Read the model definition and answer for the solid it produces. Units are mm, in the model's axes. Face numbers are marked on the shaded views. A direction names the side the tool comes from. Coordinates: 2 decimals unless noted, no trailing zeros. Write each loop counter-clockwise with the first axis right and the second up, starting at its lowest first coordinate (ties: lowest second). Pieces come first, ordered by that corner, then holes.
Item 1: Section D-D (z = 1) is taken. Give the vertices of the cut face in (x, y), then the cut area to 3 significant figures.
Item 2: Each of these flat-tipped pins is pushed along its axis until it touches: P1, Ø0.9, axis at x = -59.5, y = 28.5, coming from the +Z side; P2, Ø3, axis at x = -61.5, z = 6, coming from the -Y side; P3, Ø4, axis at x = -61.5, z = 11, coming from the -Y side. Where does it stop, or does it pass through?
Item 3: Straight lines are drawn through the part: probe 1 along Z at (x, y) = (-56.75, 27.75); probe 2 along X at (y, z) = (28.5, 3.25); probe 3 along Z at (x, y) = (-59.25, 29.5). For each, find the intervals that lie inside material, in ascending order.
Item 4: Section B-B (x = -59) is taken. Give the vertices of the cut face in (y, z), then the cut area to 3 significant figures.
Item 5: Section A-A (z = 11.75) is taken. Give the vertices of the cut face in (x, y).
Item 6: Section C-C (y = 25.5) is taken. Give the vertices of the cut face in (x, z), then the cut area to 3 significant figures.
Item 7: Determine the mould class of the marked faces 4, 5 and 6 for opening direction X: released by +X, released by -X, zero draft, split by the parting line, or undercut.
Item 8: A tool of negligible diameter and unlimited length cuts with its end or side. For the marked faces 1, 2 and 3, from which of +Z, -Z, +X, -X, +Y, -Y can it reach the whole face along a straight path? Write none if from no direction.
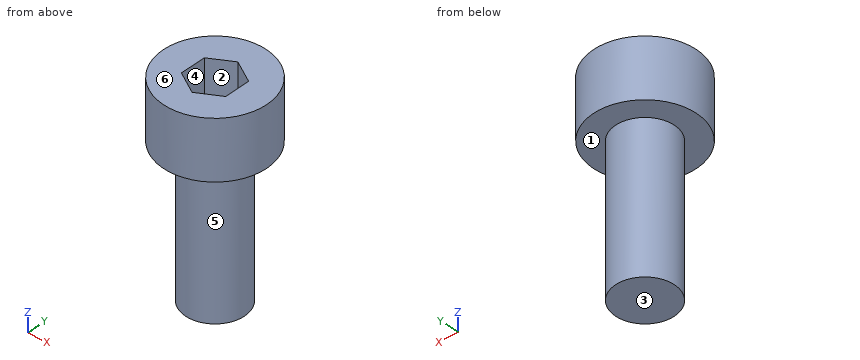
Solid Edge part; units mm, degrees
sketch "Sketch1" plane through (0, 0, 0) normal (0, 0, 1) x (1, 0, 0)
  circle A0 centre (-59.3555, 28.6102) radius 2
extrude "Protrusion1" add sketch "Sketch1" along normal blind 10
sketch "Sketch2" plane through (-59.3555, 28.6102, 10) normal (0, 0, 1) x (1, 0, 0)
  circle A0 centre (0, 0) radius 3.5
extrude "kopdia7x4" add sketch "Sketch2" along normal blind 4
cosmetic_thread "Thread1"
sketch "Sketch3" plane through (-59.3555, 28.6102, 14) normal (0, 0, 1) x (1, 0, 0)
  line L0 (-1.5, 0.866) -> (-1.5, -0.866)
  line L1 (-1.5, -0.866) -> (0, -1.7321)
  line L2 (0, -1.7321) -> (1.5, -0.866)
  line L3 (1.5, -0.866) -> (1.5, 0.866)
  line L4 (1.5, 0.866) -> (0, 1.7321)
  line L5 (0, 1.7321) -> (-1.5, 0.866)
extrude "zeskant" cut sketch "Sketch3" against normal blind 3
Established:
1. outline: circle Ø4 at (-59.36, 28.61)
1. area: 12.6 mm2
2. P1: stops at z = 11
2. P2: stops at y = 26.72
2. P3: stops at y = 25.11
3. probe 1: z = 10 to 14
3. probe 2: x = -61.35 to -57.36
3. probe 3: z = 0 to 11
4. outline: (25.13, 10) - (26.64, 10) - (26.64, 0) - (30.58, 0) - (30.58, 10) - (32.09, 10) - (32.09, 14) - (30.14, 14) - (30.14, 11) - (27.08, 11) - (27.08, 14) - (25.13, 14) - close
4. area: 58.1 mm2
5. outline: circle Ø7 at (-59.36, 28.61); hole (-60.86, 27.74) - (-59.36, 26.88) - (-57.86, 27.74) - (-57.86, 29.48) - (-59.36, 30.34) - (-60.86, 29.48) - close
6. outline: (-60.96, 10) - (-57.75, 10) - (-57.75, 14) - (-60.96, 14) - close
6. area: 12.8 mm2
7. face 4: undercut
7. face 5: split by the parting line
7. face 6: zero draft
8. face 1: -Z
8. face 2: +Z
8. face 3: -Z, +X, -X, +Y, -Y
